Design review of the part built by this model. Coordinates are the model's own, in mm. A direction names the side the tool comes from. Give positions to 0.01 mm unless a question says otherwise; leave off trailing zeros. Write each loop counter-clockwise with the first axis right and the second up, starting at its lowest first coordinate (ties: lowest second). Pieces come first, ordered by that corner, then holes. Notation, with made-up numbers: (75, -39) -> (94, -39) arc R35 cw to (94, -5) -> close; hole circle Ø4 at (49, -13.5). An arc over 180 degrees is marked (long way). Put each result on its own line as item: value. Start each with the question number.
from build123d import *

# Parameters (mm, degrees)
SCHIZZO1_W                   = 644
SCHIZZO1_H                   = 42
ESTRUSIONE_ESTRUSIONE1_DEPTH = 65
SCHIZZO2_W                   = 624
SCHIZZO2_H                   = 55
TAGLIO_ESTRUSIONE1_DEPTH     = 32
SCHIZZO4_R                   = 5.25
TAGLIO_ESTRUSIONE2_DEPTH     = 10
TAGLIO_ESTRUSIONE3_REACH     = 649.613
SCHIZZO5_R                   = 5


with BuildPart() as part:
    # Schizzo1 → Estrusione-Estrusione1 (new body)
    with BuildSketch(Plane.XY):
        Rectangle(SCHIZZO1_W, SCHIZZO1_H)
    extrude(amount=-ESTRUSIONE_ESTRUSIONE1_DEPTH)

    # Schizzo2 → Taglio-Estrusione1 (cut)
    with BuildSketch(Plane.XZ.offset(21)):
        with Locations((0, -32.5)):
            Rectangle(SCHIZZO2_W, SCHIZZO2_H)
    extrude(amount=-TAGLIO_ESTRUSIONE1_DEPTH, mode=Mode.SUBTRACT)

    # Schizzo4 → Taglio-Estrusione2 (cut)
    with BuildSketch(Plane(origin=(0, 21, -21), x_dir=(1, 0, 0), z_dir=(0, -1, 0))):
        with Locations(Location((-15, -11.5, 0), (0, 0, 180))):
            Circle(SCHIZZO4_R)
        with Locations(Location((15, -11.5, 0), (0, 0, 180))):
            Circle(SCHIZZO4_R)
    extrude(amount=TAGLIO_ESTRUSIONE2_DEPTH, mode=Mode.SUBTRACT)

    # Taglio-Estrusione3: up to this face of the body (flat: up to its plane)
    taglio_estrusione3_end = Plane(part.part.faces().sort_by_distance((-322, 0, -32.5))[0])
    # Schizzo5 → Taglio-Estrusione3 (cut, up to the picked face)
    with BuildSketch(Plane(origin=(322, 0, 0), x_dir=(0, 0, -1), z_dir=(1, 0, 0)), mode=Mode.PRIVATE) as taglio_estrusione3_sk1:
        with Locations(Location((12.5, 0, 0), (0, 0, 270))):
            Circle(SCHIZZO5_R)
    taglio_estrusione3_tool1 = split(extrude(taglio_estrusione3_sk1.sketch, amount=-TAGLIO_ESTRUSIONE3_REACH, mode=Mode.PRIVATE), bisect_by=taglio_estrusione3_end, keep=Keep.BOTH, mode=Mode.PRIVATE)
    # Schizzo5 → Taglio-Estrusione3 (cut, up to the picked face)
    with BuildSketch(Plane(origin=(322, 0, 0), x_dir=(0, 0, -1), z_dir=(1, 0, 0)), mode=Mode.PRIVATE) as taglio_estrusione3_sk2:
        with Locations(Location((52.5, 0, 0), (0, 0, 270))):
            Circle(SCHIZZO5_R)
    taglio_estrusione3_tool2 = split(extrude(taglio_estrusione3_sk2.sketch, amount=-TAGLIO_ESTRUSIONE3_REACH, mode=Mode.PRIVATE), bisect_by=taglio_estrusione3_end, keep=Keep.BOTH, mode=Mode.PRIVATE)
    add(taglio_estrusione3_tool1.solids().sort_by(Axis((322, 0, -12.5), (-1, 0, 0)))[0], mode=Mode.SUBTRACT)
    add(taglio_estrusione3_tool2.solids().sort_by(Axis((322, 0, -52.5), (-1, 0, 0)))[0], mode=Mode.SUBTRACT)


solid = part.part
Q1. Take a section at B-B on z = -32.5. Give the boundary of the cut face in (x, y).
Q2. Take a section at C-C on x = -204.5. Give the boundary of the cut face in (y, z).
Q3. For pin 1 (8.5 mm diameter, centred on x = -15, z = -32.5, fed in from -Y); pin 2 (2 mm diameter, centred on x = -257.5, z = -7.5, fed in from -Y), all flat-tipped, find the tip position at first contact; note any pin that passes through.
Q4. Machinability: for faces 1 (the face through (-316.93, 0.651, -57.457)), 2 (the face through (-312, -5, -33)), which of the approach directions +Z, -Z, +X, -X, +Y, -Y give a long, thin tool a straight path to every point of the face, cutting with its end or side? Answer none if there is none.
Q5. Mouldability with a two-part tool opening along X and no side actions: class faces 3 (the face through (-322, 0, -32)), 4 (the face through (-5, 0, -65)), 5 (the face through (-4, -5, -5)) as +X half, -X half, draft (parallel to the pull), parting line (faces both ways), or undercut.
Q6. Take a section at A-A on x = -15. Give the boundary of the cut face in (y, z).
Q7. To check wall thickness, follow probe 1 along Z at (x, y) = (318, 0); probe 2 along X at (y, z) = (18.5, -32.5); probe 3 along X at (y, z) = (-10, -19). State the ranges of each line that lie inside material, in increasing order. Write a range as from..to.
Result:
1. outline: (-322, -21) -> (-312, -21) -> (-312, 11) -> (-20.25, 11) -> (-20.25, 21) -> (-322, 21) -> close; (-9.75, 11) -> (9.75, 11) -> (9.75, 21) -> (-9.75, 21) -> close; (20.25, 11) -> (312, 11) -> (312, -21) -> (322, -21) -> (322, 21) -> (20.25, 21) -> close
2. outline: (-21, -65) -> (21, -65) -> (21, 0) -> (-21, 0) -> (-21, -5) -> (11, -5) -> (11, -60) -> (-21, -60) -> close
3. pin 1: passes through
3. pin 2: stops at y = 11
4. face 1: +X, -X
4. face 2: -Y
5. face 3: -X half
5. face 4: draft
5. face 5: undercut
6. outline: (-21, -65) -> (21, -65) -> (21, -37.75) -> (11, -37.75) -> (11, -60) -> (-21, -60) -> close; (-21, -5) -> (11, -5) -> (11, -27.25) -> (21, -27.25) -> (21, 0) -> (-21, 0) -> close
7. probe 1: z = -65..-57.5, -47.5..-17.5, -7.5..0
7. probe 2: x = -322..-20.25, -9.75..9.75, 20.25..322
7. probe 3: x = -322..-312, 312..322
